from build123d import *

# Parameters (mm, degrees)
SKETCH010_R     = 1.75
PAD005_DEPTH    = 6.5
PAD006_DEPTH    = 10
SKETCH012_R     = 3
POCKET004_DEPTH = 14.45
SKETCH013_W     = 42.25
SKETCH013_H     = 43.25
SKETCH013_R     = 19.5
SKETCH013_R_2   = 1
PAD007_DEPTH    = 5
SKETCH054_W     = 13.95
SKETCH054_H     = 1
POCKET023_DEPTH = 1


with BuildPart() as part:
    # Sketch010 → Pad005 (new body)
    with BuildSketch(Plane.XZ):
        Polygon((14.45, 10), (14.45, -10), (-14.45, -10), (-14.45, 10), (-21.125, 20.5), (-21.125, 25.5), (21.125, 25.5), (21.125, 20.5), align=None)
        with Locations((-5, 7.5)):
            Circle(SKETCH010_R, mode=Mode.SUBTRACT)
        with Locations((5, 7.5)):
            Circle(SKETCH010_R, mode=Mode.SUBTRACT)
        with Locations((-5, -7.5)):
            Circle(SKETCH010_R, mode=Mode.SUBTRACT)
        with Locations((5, -7.5)):
            Circle(SKETCH010_R, mode=Mode.SUBTRACT)
    extrude(amount=PAD005_DEPTH)

    # Sketch011 → Pad006 (join)
    with BuildSketch(Plane.XZ):
        Polygon((-21.125, 25.5), (21.125, 25.5), (21.125, 20.5), (14.45, 10), (-14.45, 10), (-21.125, 20.5), align=None)
    extrude(amount=-PAD006_DEPTH)

    # Sketch012 → Pocket004 (cut, symmetric)
    with BuildSketch(Plane.YZ):
        with Locations((5, -14.5)):
            Circle(SKETCH012_R)
    extrude(amount=POCKET004_DEPTH, both=True, mode=Mode.SUBTRACT)

    # Sketch013 (on Face9 of Pocket004) → Pad007 (join)
    with BuildSketch(Plane(origin=(0, 0, 25.5), x_dir=(-1, 0, 0), z_dir=(0, 0, 1))):
        with Locations((0, -31.625)):
            Rectangle(SKETCH013_W, SKETCH013_H)
        with Locations((0, -31.625)):
            Circle(SKETCH013_R, mode=Mode.SUBTRACT)
        with Locations((-16.25, -15.375)):
            Circle(SKETCH013_R_2, mode=Mode.SUBTRACT)
        with Locations((16.25, -15.375)):
            Circle(SKETCH013_R_2, mode=Mode.SUBTRACT)
        with Locations((16.25, -47.875)):
            Circle(SKETCH013_R_2, mode=Mode.SUBTRACT)
        with Locations((-16.25, -47.875)):
            Circle(SKETCH013_R_2, mode=Mode.SUBTRACT)
    extrude(amount=-PAD007_DEPTH)

    # Sketch054 → Pocket023 (cut)
    with BuildSketch(Plane.XZ):
        with Locations((-7.475, 0)):
            Rectangle(SKETCH054_W, SKETCH054_H)
        with Locations((7.475, 0)):
            Rectangle(SKETCH054_W, SKETCH054_H)
    extrude(amount=POCKET023_DEPTH, mode=Mode.SUBTRACT)


with BuildPart() as part_1:
    # Body003 placement: moved
    add(part.part.moved(Location((-30.55, -3.5, 0))))


solid = part_1.part
For this review, take the finished solid that the model builds, in its own axes (mm). A direction names the side the tool comes from. Round coordinates to 2 decimals unless told otherwise and drop trailing zeros. Write each loop counter-clockwise with the first axis right and the second up, starting at its lowest first coordinate (ties: lowest second). Pieces come first, ordered by that corner, then holes. Notation, with made-up numbers: (-2, 79) - (57, 79) arc R25 cw to (57, 118) - close; hole circle Ø6 at (-10.75, 89.5). An arc over 180 degrees is marked (long way). Write item = value, one per line. Start each with the question number.
1. Consider section A-A on z = -7.5. State the section outline as (x, y) points.
2. Consider section D-D on x = -14.3. State the section outline as (y, z) points (3 decimals).
3. Draft analysis for pull direction Y (two halves, no side actions). For faces 4 (the face through (-30.3, -3.5, 0.1)), 5 (the face through (-30, 1, 10)), 6 (the face through (-14.838, 43.532, 23.035)), state which applies: released by +Y, released by -Y, zero draft, split by the parting line, or undercut.
4. Consider section B-B on x = -43. State the section outline as (y, z) points, plus the area to 3 significant figures.
5. For pin 1 Ø0.5 at (y, z) = (-4, 0) entering from -X; pin 2 Ø5 at (y, z) = (-8, -4) entering from -X; pin 3 Ø3 at (x, z) = (-28.5, 15) entering from +Y, all flat-tipped, find the tip position at first contact; note any pin that passes through.
6. Wall thickness on L1, parallel to Z at x = -35.55, y = -6; L2, parallel to Z at x = -18, y = -4; L3, parallel to Y at x = -14.3, z = 23.5 (3 decimals): over which ranges is each line inside the solid? List them lowest first.
7. Consider section C-C on y = 5. State the section outline as (x, z) points (3 decimals), plus the area to 3 significant figures.
8. For faces 1 (the face through (-16.1, -7, 0)), 2 (the face through (-30, 6, 25.5)), 3 (the face through (-45, -7, 0)), list the 3-axis set-ups (+Z, -Z, +X, -X, +Y, -Y) from which the entire face can be reached by the end or side of a thin tool; tool diameter is ignored.
Evaluation:
q1.outline = (-45, -10) - (-37.3, -10) - (-37.3, -3.5) - (-45, -3.5) - close; (-33.8, -10) - (-27.3, -10) - (-27.3, -3.5) - (-33.8, -3.5) - close; (-23.8, -10) - (-16.1, -10) - (-16.1, -3.5) - (-23.8, -3.5) - close
q2.outline = (-10, 12.831) - (6.5, 12.831) - (6.5, 20.5) - (10.875, 20.5) - (10.875, 25.5) - (-10, 25.5) - close; (12.875, 20.5) - (17.346, 20.5) - (17.346, 25.5) - (12.875, 25.5) - close; (38.904, 20.5) - (43.375, 20.5) - (43.375, 25.5) - (38.904, 25.5) - close; (45.375, 20.5) - (49.75, 20.5) - (49.75, 25.5) - (45.375, 25.5) - close
q3.face_4 = released by +Y
q3.face_5 = zero draft
q3.face_6 = undercut
q4.outline = (-10, -10) - (-3.5, -10) - (-3.5, -0.5) - (-4.5, -0.5) - (-4.5, 0.5) - (-3.5, 0.5) - (-3.5, 10) - (6.5, 10) - (6.5, 20.5) - (13.12, 20.5) - (13.12, 25.5) - (-10, 25.5) - close; (43.13, 20.5) - (49.75, 20.5) - (49.75, 25.5) - (43.13, 25.5) - close
q4.area = 451 mm2
q5.pin_1 = -31.05
q5.pin_2 = -45
q5.pin_3 = 6.5
q6.L1 = -10 to -9.25, -5.75 to 5.75, 9.25 to 25.5
q6.L2 = -10 to -0.5, 0.5 to 25.5
q6.L3 = -10 to 10.875, 12.875 to 17.346, 38.904 to 43.375, 45.375 to 49.75
q7.outline = (-51.675, 20.5) - (-45, 10) - (-16.1, 10) - (-9.425, 20.5) - (-9.425, 25.5) - (-51.675, 25.5) - close
q7.area = 585 mm2
q8.face_1 = -Z, +X, +Y, -Y
q8.face_2 = +Z, +X, -X, +Y, -Y
q8.face_3 = -Z, -X, +Y, -Y
